Verification items for the finished model (mm, model axes). Round coordinates to 2 decimals unless told otherwise and drop trailing zeros. Order: outer loops, then holes, each group sorted by start corner. A loop starts at its lowest first (then second) coordinate and runs counter-clockwise, first axis right, second up. Notation, with made-up numbers: M -24.5,65 L 29.5,65 A31 cw 29.5,98 Z; hole C 41.5,53 d10. An arc over 180 degrees is marked long. Use CSV: the item, a comma, the result in double quotes. Start each with the question number.
Q1. Sectioned sample at B-B (y = 23.15). Enter the section's corners in (x, z).
Q2. Scan lines: line 1 (Y direction, x = -33.15, z = 16.5); line 2 (X direction, y = -23.15, z = 16.75). Record each from-to range of solid material in increasing order.
Q3. Sectioned sample at A-A (x = 33.15). Enter the section's corners in (y, z), and give its area (3 significant figures).
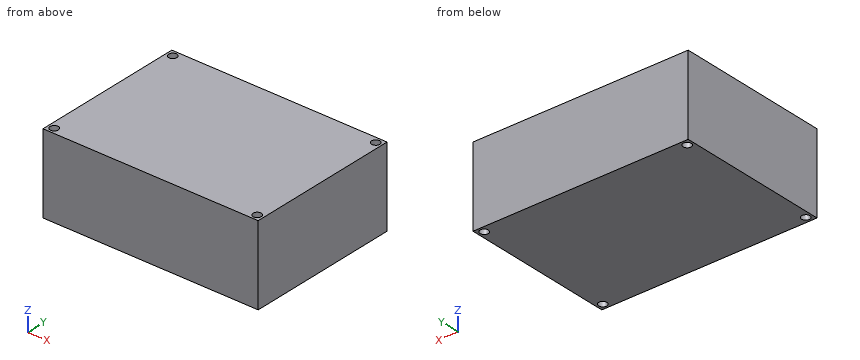
```python
from build123d import *

# Parameters (mm, degrees)
SKETCH_W                = 70.3
SKETCH_H                = 50.3
PAD_DEPTH               = 26
SKETCH001_R             = 1.35
POCKET_DEPTH            = 206.53554
SKETCH001_MIRRORED_2_R  = 1.35
POCKET_MIRRORED_2_DEPTH = 206.53554


with BuildPart() as part:
    # Sketch → Pad (new body)
    with BuildSketch(Plane.XY):
        Rectangle(SKETCH_W, SKETCH_H)
    extrude(amount=PAD_DEPTH)

    # Sketch001 → Pocket (cut, through all)
    with BuildSketch(Plane.XY):
        with Locations((33.15, 23.15)):
            Circle(SKETCH001_R)
    pocket = extrude(amount=POCKET_DEPTH, mode=Mode.SUBTRACT)

    # Sketch001 Mirrored 2 → Pocket Mirrored 2 (cut, through all)
    with BuildSketch(Plane(origin=(0, 0, 0), x_dir=(-1, 0, 0), z_dir=(0, 0, -1))):
        with Locations((33.15, 23.15)):
            Circle(SKETCH001_MIRRORED_2_R)
    pocket_mirrored_2 = extrude(amount=-POCKET_MIRRORED_2_DEPTH, mode=Mode.SUBTRACT)

    # Mirrored001: Pocket, Pocket Mirrored 2 across Sketch001 H_Axis
    add(pocket.mirror(Plane.ZX), mode=Mode.SUBTRACT)
    add(pocket_mirrored_2.mirror(Plane.ZX), mode=Mode.SUBTRACT)


solid = part.part
```
Verdict:
1,outline,"M -35.15,0 L -34.5,0 L -34.5,26 L -35.15,26 Z; M -31.8,0 L 31.8,0 L 31.8,26 L -31.8,26 Z; M 34.5,0 L 35.15,0 L 35.15,26 L 34.5,26 Z"
2,line 1,"y = -25.15 to -24.5, -21.8 to 21.8, 24.5 to 25.15"
2,line 2,"x = -35.15 to -34.5, -31.8 to 31.8, 34.5 to 35.15"
3,outline,"M -25.15,0 L -24.5,0 L -24.5,26 L -25.15,26 Z; M -21.8,0 L 21.8,0 L 21.8,26 L -21.8,26 Z; M 24.5,0 L 25.15,0 L 25.15,26 L 24.5,26 Z"
3,area,"1,170 mm²"
